Autodesk Fusion 360 part; units mm, degrees
sketch "Sketch1" plane through (0, 0, 0) normal (0, 0, 1) x (1, 0, 0)
  line L0 (0, 0) -> (70.5, 0)
  line L1 (70.5, 0) -> (70.5, 32)
  line L2 (70.5, 32) -> (0, 32)
  line L3 (0, 32) -> (0, 0)
  dimension "d1" = 70.5
  dimension "d2" = 32
extrude "Extrude1" add sketch "Sketch1" along normal blind 1.5
extrude "Extrude2" add 1 faces at (47, 32, 0.5) along direction (0, 1, 0) blind 1
extrude "Extrude3" add 1 faces at (23.5, 22, 1.5) along direction (0, 0, 1) blind 2
sketch "Sketch2" plane through (0, 0, 3.5) normal (0, 0, 1) x (-1, 0, 0)
  line L0 (0, -33) -> (0, 0)
  line L1 (0, 0) -> (-70.5, 0)
  line L2 (-70.5, 0) -> (-70.5, -33)
  line L3 (-70.5, -33) -> (0, -33)
  line L4 (-35.25, -33) -> (-35.25, -31)
  line L5 (-35.25, -31) -> (-35.25, -28.75)
  line L6 (-60.25, -26.5) -> (-10.25, -26.5)
  line L7 (-10.25, -26.5) -> (-10.25, -31)
  line L8 (-10.25, -31) -> (-60.25, -31)
  line L9 (-60.25, -31) -> (-60.25, -26.5)
  line L10 (-60.25, -26.5) -> (-10.25, -31) construction
  line L11 (-10.25, -26.5) -> (-60.25, -31) construction
  point P0 (-35.25, -28.75)
  dimension "d9" = 2
  dimension "d10" = 2.25
  dimension "d11" = 50
  dimension "d12" = 4.5
extrude "Extrude4" cut sketch "Sketch2" against normal blind 2.2 contours L6 L7 L8 L9
extrude "Extrude5" cut 1 faces at (43.5833, 26.5, 2.7667) along direction (0, -1, 0) blind 0.7
extrude "Extrude6" cut 1 faces at (10.25, 27.5333, 2.7667) along direction (-1, 0, 0) blind 0.35
extrude "Extrude7" cut 1 faces at (60.25, 27.5333, 2.0333) along direction (1, 0, 0) blind 0.35
extrude "Extrude8" add 1 faces at (0, 22, 2.3333) along direction (-1, 0, 0) blind 1.5
extrude "Extrude9" add 1 faces at (22.5, 33, 1.1667) along direction (0, 1, 0) blind 1
extrude "Extrude10" add 1 faces at (46.5, 0, 1.1667) along direction (0, -1, 0) blind 1
sketch "Sketch3" plane through (0, 0, 3.5) normal (0, 0, 1) x (-1, 0, 0)
  line L0 (-60.6, -25.8) -> (-9.9, -25.8)
  line L1 (-9.9, -25.8) -> (-9.9, -31)
  line L2 (-9.9, -31) -> (-60.6, -31)
  line L3 (-60.6, -31) -> (-60.6, -25.8)
  line L4 (-70.5, 1) -> (-70.5, -34)
  line L5 (-70.5, -34) -> (1.5, -34)
  line L6 (1.5, -34) -> (1.5, 1)
  line L7 (1.5, 1) -> (-70.5, 1)
  line L8 (-10, -15) -> (-25, -15)
  line L9 (-25, -15) -> (-25, -3)
  line L10 (-25, -3) -> (-10, -3)
  line L11 (-10, -3) -> (-10, -15)
extrude "Extrude11" cut sketch "Sketch3" against normal blind 0.7 contours L8 L9 L10 L11
sketch "Sketch4" plane through (0, 0, 3.5) normal (0, 0, 1) x (-1, 0, 0)
  line L0 (-25, -15) -> (-25, -3)
  line L1 (-25, -3) -> (-10, -3)
  line L2 (-10, -3) -> (-10, -15)
  line L3 (-10, -15) -> (-25, -15)
  line L4 (-60.6, -25.8) -> (-9.9, -25.8)
  line L5 (-9.9, -25.8) -> (-9.9, -31)
  line L6 (-9.9, -31) -> (-60.6, -31)
  line L7 (-60.6, -31) -> (-60.6, -25.8)
  line L8 (-70.5, 1) -> (-70.5, -34)
  line L9 (-70.5, -34) -> (1.5, -34)
  line L10 (1.5, -34) -> (1.5, 1)
  line L11 (1.5, 1) -> (-70.5, 1)
  line L12 (1.5, -34) -> (-70.5, -34)
  line L13 (-70.5, -34) -> (-70.5, -33)
  line L14 (-70.5, -33) -> (1.5, -33)
  line L15 (1.5, -33) -> (1.5, -34)
  line L16 (1.5, 1) -> (0.5, 1)
  line L17 (0.5, 1) -> (0.5, -34)
  line L18 (0.5, -34) -> (1.5, -34)
  line L19 (1.5, -34) -> (1.5, 1)
  line L20 (1.5, 1) -> (-70.5, 1)
  line L21 (-70.5, 1) -> (-70.5, 0)
  line L22 (-70.5, 0) -> (1.5, 0)
  line L23 (1.5, 0) -> (1.5, 1)
  line L24 (-70.5, -34) -> (-69.5, -34)
  line L25 (-69.5, -34) -> (-69.5, 1)
  line L26 (-69.5, 1) -> (-70.5, 1)
  line L27 (-70.5, 1) -> (-70.5, -34)
  dimension "d29" = 1
  dimension "d30" = 1
  dimension "d31" = 1
  dimension "d32" = 1
extrude "Extrude12" add sketch "Sketch4" along normal blind 4 contours L8 L11 L20 L21 L22 L25 L26 L27 | L8 L14 L22 L25 L27 | L11 L17 L20 L22 L25 | L8 L9 L12 L13 L14 L24 L25 L27 | L10 L11 L16 L17 L19 L20 L22 L23 | L9 L12 L14 L17 L25 | L10 L14 L17 L19 L22 | L9 L10 L12 L14 L15 L17 L18 L19
sketch "Sketch5" plane through (0, 0, 3.5) normal (0, 0, 1) x (-1, 0, 0)
  line L0 (-69.5, -33) -> (0.5, -33)
  line L1 (0.5, -33) -> (0.5, 0)
  line L2 (0.5, 0) -> (-69.5, 0)
  line L3 (-69.5, 0) -> (-69.5, -33)
  line L4 (-25, -15) -> (-25, -3)
  line L5 (-25, -3) -> (-10, -3)
  line L6 (-10, -3) -> (-10, -15)
  line L7 (-10, -15) -> (-25, -15)
  line L8 (-60.6, -25.8) -> (-9.9, -25.8)
  line L9 (-9.9, -25.8) -> (-9.9, -31)
  line L10 (-9.9, -31) -> (-60.6, -31)
  line L11 (-60.6, -31) -> (-60.6, -25.8)
  line L12 (-70.5579, -29.7) -> (-66.2579, -29.7)
  circle A0 centre (-66.2579, -29.7) radius 1.375
  line L13 (-2, -34) -> (-2, -29.7)
  line L14 (1.461, -29.9433) -> (-5.539, -29.9433)
  circle A1 centre (-5.539, -29.9433) radius 1.375
  dimension "d36" = 4.3
  dimension "d37" = 2.75
  dimension "d38" = 4.3
  dimension "d39" = 7
  dimension "d40" = 2.75
extrude "Extrude13" add sketch "Sketch5" along normal blind 5 contours A1 | A0
sketch "Sketch6" plane through (0, -1, 0) normal (0, -1, 0) x (1, 0, 0)
  line L0 (-1.5, 0) -> (70.5, 0)
  line L1 (70.5, 0) -> (70.5, 7.5)
  line L2 (70.5, 7.5) -> (-1.5, 7.5)
  line L3 (-1.5, 7.5) -> (-1.5, 0)
  line L4 (70.5, 6.1254) -> (49.5, 6.1254)
  line L5 (49.5, 6.1254) -> (42.1, 6.1254)
  line L6 (42.1, 6.1254) -> (42.1, 7.5)
  line L7 (42.1, 7.5) -> (42.1, 8)
  line L8 (42.1, 8) -> (49.5, 8)
  line L9 (42.1, 8) -> (49.5, 8)
  line L10 (49.5, 8) -> (49.5, 5)
  line L11 (49.5, 5) -> (42.1, 5)
  line L12 (42.1, 5) -> (42.1, 8)
  dimension "d43" = 21
  dimension "d44" = 7.4
  dimension "d45" = 0.5
  dimension "d46" = 3
extrude "Extrude14" cut sketch "Sketch6" against normal blind 1 contours L2 L7 L8 L9 L10 L12 | L2 L5 L6 L10 L12 | L5 L10 L11 L12
sketch "Sketch7" plane through (0, 0, 3.5) normal (0, 0, 1) x (-1, 0, 0)
  circle A0 centre (-66.2579, -29.7) radius 1.375
  circle A1 centre (-5.539, -29.9433) radius 1.375
  line L0 (-69.5, -33) -> (0.5, -33)
  line L1 (0.5, -33) -> (0.5, 0)
  line L2 (0.5, 0) -> (-69.5, 0)
  line L3 (-69.5, 0) -> (-69.5, -33)
  line L4 (-25, -15) -> (-25, -3)
  line L5 (-25, -3) -> (-10, -3)
  line L6 (-10, -3) -> (-10, -15)
  line L7 (-10, -15) -> (-25, -15)
  line L8 (-60.6, -25.8) -> (-9.9, -25.8)
  line L9 (-9.9, -25.8) -> (-9.9, -31)
  line L10 (-9.9, -31) -> (-60.6, -31)
  line L11 (-60.6, -31) -> (-60.6, -25.8)
  line L12 (-66.2579, -29.7) -> (-66.2579, -6.5)
  circle A2 centre (-66.2579, -6.5) radius 1.375
  line L13 (-5.539, -29.9433) -> (-5.539, -6.7433)
  circle A3 centre (-5.539, -6.7433) radius 1.375
  dimension "d49" = 23.2
  dimension "d50" = 2.75
  dimension "d51" = 23.2
  dimension "d52" = 2.75
extrude "Extrude15" add sketch "Sketch7" along normal blind 5 contours A2 | A3
extrude "Extrude16" cut 2 faces at (66.7302, 30.022, 8.5) (66.8634, 6.1681, 8.5) along direction (0, 0, -1) blind 5
extrude "Extrude17" cut 2 faces at (5.5048, 28.9699, 8.5) (5.4119, 6.9636, 8.5) along direction (0, 0, -1) blind 5
sketch "Sketch8" plane through (0, 0, 3.5) normal (0, 0, 1) x (-1, 0, 0)
  line L0 (-69.5, -33) -> (0.5, -33)
  line L1 (0.5, -33) -> (0.5, 0)
  line L2 (0.5, 0) -> (-69.5, 0)
  line L3 (-69.5, 0) -> (-69.5, -33)
  line L4 (-25, -15) -> (-25, -3)
  line L5 (-25, -3) -> (-10, -3)
  line L6 (-10, -3) -> (-10, -15)
  line L7 (-10, -15) -> (-25, -15)
  line L8 (-60.6, -25.8) -> (-9.9, -25.8)
  line L9 (-9.9, -25.8) -> (-9.9, -31)
  line L10 (-9.9, -31) -> (-60.6, -31)
  line L11 (-60.6, -31) -> (-60.6, -25.8)
  line L12 (-70.5, -34) -> (-70.5, -28.2)
  line L13 (-70.5, -28.2) -> (-66.5, -28.2)
  line L14 (-70.5, -34) -> (-64.7, -34)
  line L15 (-64.7, -34) -> (-64.7, -30)
  line L16 (-64.7, -30) -> (-64.7, -27.5)
  line L17 (-66.5, -28.2) -> (-64.7, -28.2)
  circle A0 centre (-64.7, -28.2) radius 1.25
  line L18 (-64.7, -28.2) -> (-64.7, -26.95)
  line L19 (-64.7, -26.95) -> (-64.7, -6.95)
  circle A1 centre (-64.7, -5.7) radius 1.25
  line L20 (-64.7, -5.7) -> (-8.25, -5.7)
  circle A2 centre (-7, -5.7) radius 1.25
  line L21 (-7, -5.7) -> (-7, -26.95)
  circle A3 centre (-7, -28.2) radius 1.25
  dimension "d72" = 5.8
  dimension "d74" = 4
  dimension "d75" = 5.8
  dimension "d76" = 4
  dimension "d77" = 2.5
  dimension "d78" = 1.25
  dimension "d79" = 20
  dimension "d80" = 2.5
  dimension "d81" = 56.45
  dimension "d82" = 2.5
  dimension "d83" = 21.25
  dimension "d84" = 2.5
extrude "Extrude18" add sketch "Sketch8" along normal blind 3 contours A3 | A2 | A1 | L16 L17 A0 | L16 A0 L18 | L16 L17 A0 L18
sketch "Sketch9" plane through (0, 0, 6.5) normal (0, 0, 1) x (-1, 0, 0)
  circle A0 centre (-64.7, -28.2) radius 1.25
extrude "Extrude19" cut 2 faces at (6.88, 5.4166, 6.5) (64.5007, 5.6393, 6.5) along direction (0, 0, -1) blind 3
sketch "Sketch10" plane through (0, 0, 3.5) normal (0, 0, 1) x (-1, 0, 0)
  circle A0 centre (-64.7, -28.2) radius 1.25
  circle A1 centre (-7, -28.2) radius 1.25
  line L0 (-69.5, -33) -> (0.5, -33)
  line L1 (0.5, -33) -> (0.5, 0)
  line L2 (0.5, 0) -> (-69.5, 0)
  line L3 (-69.5, 0) -> (-69.5, -33)
  line L4 (-25, -15) -> (-25, -3)
  line L5 (-25, -3) -> (-10, -3)
  line L6 (-10, -3) -> (-10, -15)
  line L7 (-10, -15) -> (-25, -15)
  line L8 (-60.6, -25.8) -> (-9.9, -25.8)
  line L9 (-9.9, -25.8) -> (-9.9, -31)
  line L10 (-9.9, -31) -> (-60.6, -31)
  line L11 (-60.6, -31) -> (-60.6, -25.8)
  line L12 (-64.7, -28.2) -> (-64.7, -26.95)
  line L13 (-64.7, -26.95) -> (-64.7, -6.55)
  circle A2 centre (-64.7, -5.3) radius 1.25
  line L14 (-64.7, -5.3) -> (-63.45, -5.3)
  line L15 (-63.45, -5.3) -> (-8.25, -5.3)
  circle A3 centre (-7, -5.3) radius 1.25
  dimension "d89" = 20.4
  dimension "d90" = 2.5
  dimension "d91" = 55.2
  dimension "d92" = 2.5
extrude "Extrude20" add sketch "Sketch10" along normal blind 3 contours A3 | A2
Here's how the part is built. I have some questions about the finished solid (model axes, mm). A direction names the side the tool comes from. Give positions to 0.01 mm unless a question says otherwise; leave off trailing zeros. Loops run counter-clockwise (first coordinate to the right, second up) from the corner with the lowest first, then second, coordinate; pieces in that order, holes last. Notation, with made-up numbers: (69.25, -31.5) -> (126.25, -31.5) arc R22 ccw to (126.25, -25.5) -> close; hole circle Ø9 at (26, 28). An arc over 180 degrees is marked (long way). Use one line per item in the form item = value. Start each with the question number.
1) Imagine slicing it at D-D (y = 28.2). Please give me the cut outline in (x, z).
2) Thinking about a two-plate mould opening in Y: for faces 1 (the face through (35, 34, 4)), 2 (the face through (69.5, 17, 5)), 3 (the face through (70.5, 17, 4)), which applies, +Y half, -Y half, draft (parallel to the pull), parting line (faces both ways), or undercut?
3) Imagine slicing it at A-A (z = 4.25). Please give me the cut outline in (x, y).
4) Imagine slicing it at B-B (y = 5.3). Please give me the cut outline in (x, z), then the cut area to 4 significant figures.
5) For P1, Ø2, axis at x = 7, y = 28, coming from the +Z side; P2, Ø10, axis at x = 27, y = 23, coming from the -Z side; P3, Ø3, axis at x = 50, y = 12.5, coming from the +Z side, each with a flat end and sliding along its axis, tell me the tip position at first contact or that it passes through.
6) Please list where these lines run through material, in increasing order: line 1 along Y through (x, z) = (24.5, 3); line 2 along Y through (x, z) = (25.5, 1.75); line 3 along Y through (x, z) = (51.5, 4.25).
7) Which directions (+Z, -Z, +X, -X, +Y, -Y) give clear straight access to the entire face, cutting with the end or side of a thin tool? Please do faces 4 (the face through (34.7, 33.3, 7.5)), 5 (the face through (7, 28, 6.5)).
8) Imagine slicing it at C-C (x = 7). Please give me the cut outline in (y, z).
Check values:
q1.outline = (-1.5, 0) -> (70.5, 0) -> (70.5, 7.5) -> (69.5, 7.5) -> (69.5, 3.5) -> (65.95, 3.5) -> (65.95, 6.5) -> (63.45, 6.5) -> (63.45, 3.5) -> (60.6, 3.5) -> (60.6, 1.3) -> (9.9, 1.3) -> (9.9, 3.5) -> (8.25, 3.5) -> (8.25, 6.5) -> (5.75, 6.5) -> (5.75, 3.5) -> (-0.5, 3.5) -> (-0.5, 7.5) -> (-1.5, 7.5) -> close
q2.face_1 = +Y half
q2.face_2 = undercut
q2.face_3 = draft
q3.outline = (-1.5, -1) -> (70.5, -1) -> (70.5, 34) -> (-1.5, 34) -> close; circle Ø2.5 at (7, 5.3); circle Ø2.5 at (7, 28.2); circle Ø2.5 at (64.7, 5.3); circle Ø2.5 at (64.7, 28.2); hole (-0.5, 0) -> (69.5, 0) -> (69.5, 33) -> (-0.5, 33) -> close
q4.outline = (-1.5, 0) -> (70.5, 0) -> (70.5, 7.5) -> (69.5, 7.5) -> (69.5, 3.5) -> (65.95, 3.5) -> (65.95, 6.5) -> (63.45, 6.5) -> (63.45, 3.5) -> (25, 3.5) -> (25, 2.8) -> (10, 2.8) -> (10, 3.5) -> (8.25, 3.5) -> (8.25, 6.5) -> (5.75, 6.5) -> (5.75, 3.5) -> (-0.5, 3.5) -> (-0.5, 7.5) -> (-1.5, 7.5) -> close
q4.area = 264.5 mm^2
q5.P1 = 6.5
q5.P2 = 0
q5.P3 = 3.5
q6.line_1 = -1 to 3, 15 to 25.8, 31 to 34
q6.line_2 = -1 to 25.8, 31 to 34
q6.line_3 = -1 to 0, 33 to 34
q7.face_4 = +Z, +X, -X, +Y, -Y
q7.face_5 = +Z
q8.outline = (-1, 0) -> (34, 0) -> (34, 7.5) -> (33, 7.5) -> (33, 3.5) -> (29.45, 3.5) -> (29.45, 6.5) -> (26.95, 6.5) -> (26.95, 3.5) -> (6.55, 3.5) -> (6.55, 6.5) -> (4.05, 6.5) -> (4.05, 3.5) -> (0, 3.5) -> (0, 7.5) -> (-1, 7.5) -> close
